For this review, take the finished solid that the model builds, in its own axes (mm). Face numbers are marked on the shaded views. A direction names the side the tool comes from. Round coordinates to 2 decimals unless told otherwise and drop trailing zeros. Write each loop counter-clockwise with the first axis right and the second up, starting at its lowest first coordinate (ties: lowest second). Pieces come first, ordered by that corner, then holes. Notation, with made-up numbers: (-1.75, 28) - (34.25, 28) arc R18 ccw to (34.25, 45) - close; hole circle Ø6 at (13.25, -34.5). An arc over 180 degrees is marked (long way). Answer in a Markdown table with one row per item. Add a question column.
from build123d import *

# Parameters (mm, degrees)
F1_DEPTH = 300
F2_R     = 3
F3_DEPTH = 50.801


with BuildPart() as f1:
    # F0 (on Front) → F1 (new body)
    with BuildSketch(Plane.XZ):
        Polygon((0, 50.8), (0, 0), (50.8, 0), (50.8, 1.59), (1.59, 1.59), (1.59, 50.8), align=None)
    extrude(amount=F1_DEPTH)

    # F2 (on Top) → F3 (cut, through all)
    with BuildSketch(Plane.XY):
        with Locations((9.525, -9.525)):
            Circle(F2_R)
        with Locations((9.525, -240.475)):
            Circle(F2_R)
    extrude(amount=F3_DEPTH, mode=Mode.SUBTRACT)


solid = f1.part
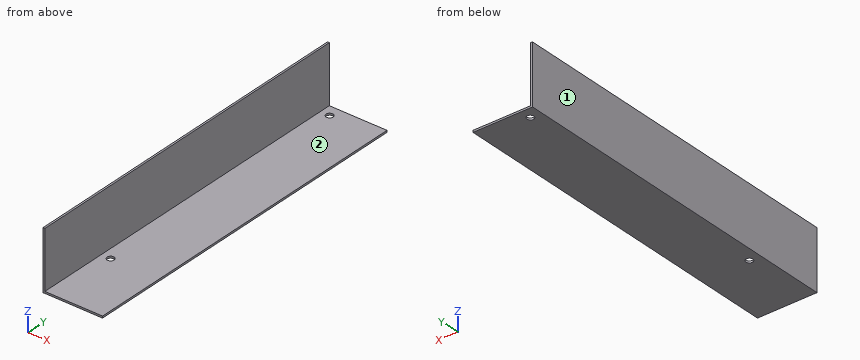
Q1. Add section B-B on z = 13. State the section outline as (x, y) points, then the cut area to 3 significant figures.
Q2. Tool access review of the marked faces 1 and 2: name each direction out of +Z, -Z, +X, -X, +Y, -Y from which nothing blocks a thin tool from reaching the whole face with its end or side.
Q3. Insertion check: pin 1 Ø6 at (x, y) = (32.5, -91) entering from +Z; pin 2 Ø15 at (y, z) = (-91.5, 36.5) entering from +X; pin 3 Ø5 at (x, y) = (9.525, -240.475) entering from -Z. Each pin has a flat end and moves straight along its axis. Give the tip position at first contact, or say it passes through.
Q4. To check wall thickness, follow probe 1 along X at (y, z) = (-15, 5.5). State the ranges of the line that lie inside material, in increasing order.
Q5. Add section A-A on x = 9. State the section outline as (y, z) points.
Q6. Add section D-D on x = 21. State the section outline as (y, z) points.
Q7. Add section C-C on y = -131. State the section outline as (x, z) points.
Answer sheet:
| question | item | result |
|---|---|---|
| 1 | outline | (0, -300) - (1.59, -300) - (1.59, 0) - (0, 0) - close |
| 1 | area | 477 mm² |
| 2 | face 1 | +Z, -Z, -X, +Y, -Y |
| 2 | face 2 | +Z, +X, +Y, -Y |
| 3 | pin 1 | stops at z = 1.59 |
| 3 | pin 2 | stops at x = 1.59 |
| 3 | pin 3 | passes through |
| 4 | probe 1 | x = 0 to 1.59 |
| 5 | outline | (-300, 0) - (-243.43, 0) - (-243.43, 1.59) - (-300, 1.59) - close; (-237.52, 0) - (-12.48, 0) - (-12.48, 1.59) - (-237.52, 1.59) - close; (-6.57, 0) - (0, 0) - (0, 1.59) - (-6.57, 1.59) - close |
| 6 | outline | (-300, 0) - (0, 0) - (0, 1.59) - (-300, 1.59) - close |
| 7 | outline | (0, 0) - (50.8, 0) - (50.8, 1.59) - (1.59, 1.59) - (1.59, 50.8) - (0, 50.8) - close |
